Part model, mm, in its own coordinate system. Give positions to 0.01 mm unless a question says otherwise; leave off trailing zeros. Loops run counter-clockwise (first coordinate to the right, second up) from the corner with the lowest first, then second, coordinate; pieces in that order, holes last. Notation, with made-up numbers: M 38,46.5 L 73,46.5 A22 ccw 73,76.5 Z; hole C 13.25,-39.75 d5. An arc over 180 degrees is marked long. Answer in a Markdown table with one row per item.
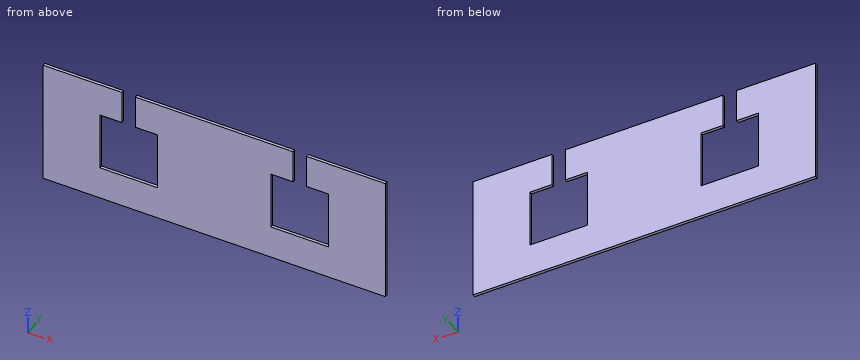
from build123d import *

# Parameters (mm, degrees)
SKETCH1_W           = 113
SKETCH1_H           = 40.6
BOSS_EXTRUDE1_DEPTH = 1
CUT_EXTRUDE1_DEPTH  = 121.076475631


with BuildPart() as part:
    # Sketch1 → Boss-Extrude1 (new body)
    with BuildSketch(Plane(origin=(0, 0, 0), x_dir=(1, 0, 0), z_dir=(0, 1, 0))):
        with Locations((56.5, 20.3)):
            Rectangle(SKETCH1_W, SKETCH1_H)
    extrude(amount=BOSS_EXTRUDE1_DEPTH)

    # Sketch2 → Cut-Extrude1 (cut, through all)
    with BuildSketch(Plane(origin=(0, 1, 0), x_dir=(1, 0, 0), z_dir=(0, 1, 0))):
        Polygon((37.75, 10.8), (30.5, 10.8), (30.5, 0), (26, 0), (26, 10.8), (18.75, 10.8), (18.75, 29.8), (37.75, 29.8), align=None)
    cut_extrude1 = extrude(amount=-CUT_EXTRUDE1_DEPTH, mode=Mode.SUBTRACT)

    # Mirror1: Cut-Extrude1 across plane
    add(cut_extrude1.mirror(Plane.ZY.offset(-56.5)), mode=Mode.SUBTRACT)


solid = part.part
(1) Saw through at B-B (z = -7). Write the cut outline in (x, y), plus the area to 3 significant figures.
Recorded:
| item | result |
|---|---|
| outline | M 0,0 L 26,0 L 26,1 L 0,1 Z; M 30.5,0 L 82.5,0 L 82.5,1 L 30.5,1 Z; M 87,0 L 113,0 L 113,1 L 87,1 Z |
| area | 104 mm^2 |
(2) Saw through at C-C (y = 0.6). Write the cut outline in (x, z).
Recorded:
| item | result |
|---|---|
| outline | M 0,-40.6 L 113,-40.6 L 113,0 L 87,0 L 87,-10.8 L 94.25,-10.8 L 94.25,-29.8 L 75.25,-29.8 L 75.25,-10.8 L 82.5,-10.8 L 82.5,0 L 30.5,0 L 30.5,-10.8 L 37.75,-10.8 L 37.75,-29.8 L 18.75,-29.8 L 18.75,-10.8 L 26,-10.8 L 26,0 L 0,0 Z |
(3) Saw through at A-A (x = 34). Write the cut outline in (y, z), plus the area to 3 significant figures.
Recorded:
| item | result |
|---|---|
| outline | M 0,-40.6 L 1,-40.6 L 1,-29.8 L 0,-29.8 Z; M 0,-10.8 L 1,-10.8 L 1,0 L 0,0 Z |
| area | 21.6 mm^2 |
(4) Saw through at D-D (z = -27.5). Write the cut outline in (x, y).
Recorded:
| item | result |
|---|---|
| outline | M 0,0 L 18.75,0 L 18.75,1 L 0,1 Z; M 37.75,0 L 75.25,0 L 75.25,1 L 37.75,1 Z; M 94.25,0 L 113,0 L 113,1 L 94.25,1 Z |
(5) Drill centre lines: line 1 along X through (y, z) = (0.4, -25.5); line 2 along X through (y, z) = (0.2, -3); line 3 along Z through (x, y) = (20, 0.65). Where is each one in solid material? Low to high.
Recorded:
| item | result |
|---|---|
| line 1 | x = 0 to 18.75, 37.75 to 75.25, 94.25 to 113 |
| line 2 | x = 0 to 26, 30.5 to 82.5, 87 to 113 |
| line 3 | z = -40.6 to -29.8, -10.8 to 0 |
